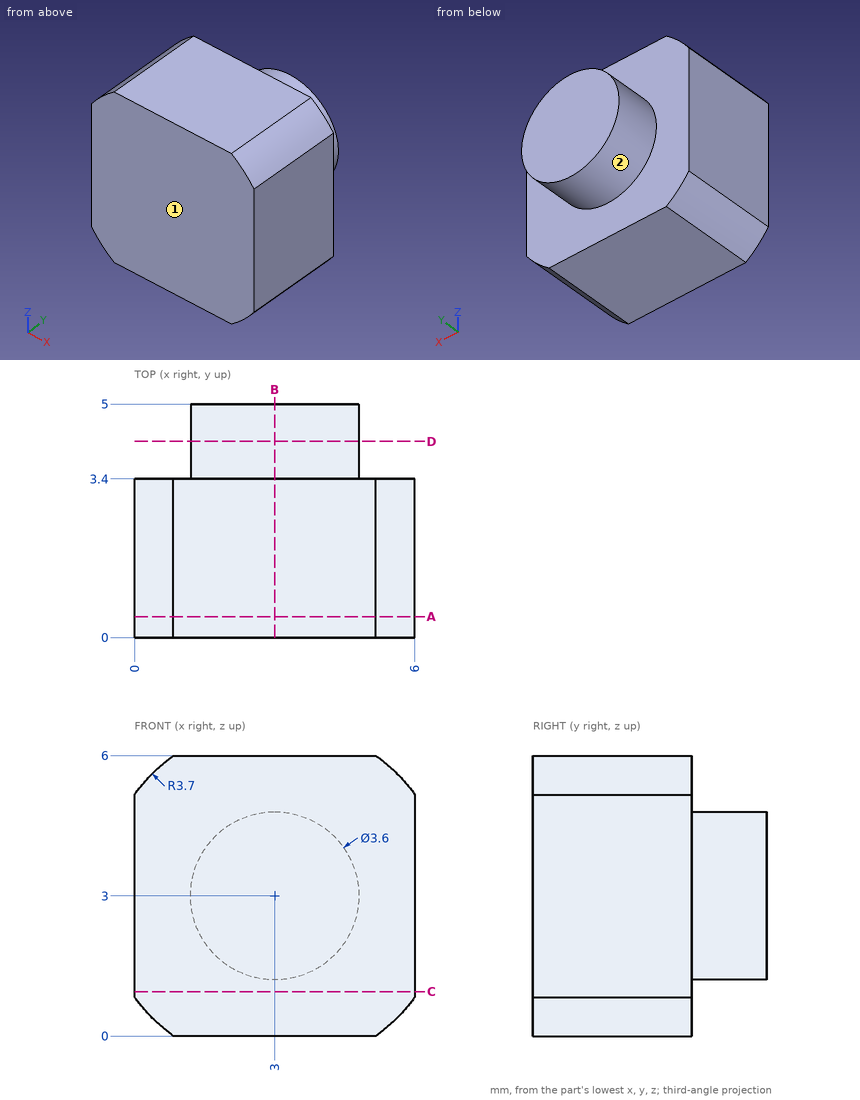
Could you check a few things on this drawing? It's one solid part, dimensions in mm from its lowest x, y, z. A direction names the side the tool comes from. Coordinates: 2 decimals unless noted, no trailing zeros. Order: outer loops, then holes, each group sorted by start corner. A loop starts at its lowest first (then second) coordinate and runs counter-clockwise, first axis right, second up. Notation, with made-up numbers: (22, 37) - (51, 37) arc R20 ccw to (51, 43) - close; hole circle Ø11 at (17.25, -25). An arc over 180 degrees is marked (long way). Answer as a JSON object with one key per item and string values. Group by question number.
Q1. I need wall thicknesses on line 1 (Y direction, x = 1.5, z = 5.75); line 2 (Z direction, x = 4.3, y = 4.15); line 3 (X direction, y = 1.3, z = 5.3). Which ranges of each line are inside material? Lowest first, please. Write a range as from..to.
Q2. On a 3-axis mill with a long thin cutter (end or side, diameter ignored), from which of +Z, -Z, +X, -X, +Y, -Y can I reach the whole of each face in a straight line? I mean the marked faces 1 and 2. Say none if no direction works.
Q3. Imagine slicing it at B-B (x = 3). Please give me the cut outline in (y, z).
Q4. Imagine slicing it at D-D (y = 4.2). Please give me the cut outline in (x, z).
Q5. Imagine slicing it at C-C (z = 0.95). Please give me the cut outline in (x, y), and give its area (3 significant figures).
Q6. Imagine slicing it at A-A (y = 0.45). Please give me the cut outline in (x, z).
Determined:
{
 "1": {"line 1": "y = 0..3.4", "line 2": "z = 1.76..4.24", "line 3": "x = 0.1..5.9"},
 "2": {"face 1": "+Z, -Z, +X, -X, -Y", "face 2": "+Y"},
 "3": {"outline": "(0, 0) - (3.4, 0) - (3.4, 1.2) - (5, 1.2) - (5, 4.8) - (3.4, 4.8) - (3.4, 6) - (0, 6) - close"},
 "4": {"outline": "circle Ø3.6 at (3, 3)"},
 "5": {"outline": "(0, 0) - (6, 0) - (6, 3.4) - (0, 3.4) - close", "area": "20.4 mm2"},
 "6": {"outline": "(0, 0.83) arc R3.7 ccw to (0.83, 0) - (5.17, 0) arc R3.7 ccw to (6, 0.83) - (6, 5.17) arc R3.7 ccw to (5.17, 6) - (0.83, 6) arc R3.7 ccw to (0, 5.17) - close"}
}
